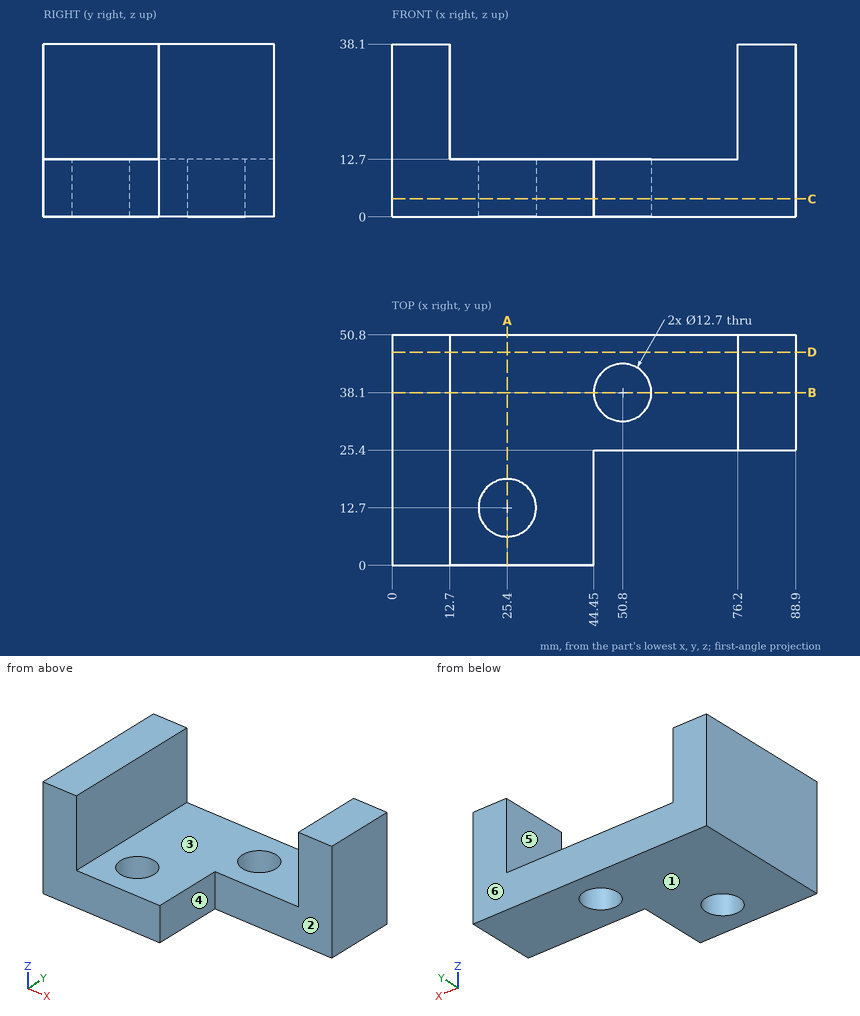
Job drawing, mm, ordinate dimensions from the low corner. One solid piece. A direction names the side the tool comes from. Coordinates: 2 decimals unless noted, no trailing zeros. Order: outer loops, then holes, each group sorted by start corner. A loop starts at its lowest first (then second) coordinate and runs counter-clockwise, first axis right, second up. Notation, with made-up numbers: (-11, 45) -> (32, 45) arc R11 cw to (32, 60) -> close; hole circle Ø8 at (30, -28.5). An arc over 180 degrees is marked (long way). Answer in a Markdown table with one row per item. Add a question column.
Q1. Band-saw the part on B-B, the plane y = 38.1. List the corners of the cut face in (x, z), then the cut area to 3 significant figures.
Q2. Band-saw the part on D-D, the plane y = 47. List the corners of the cut face in (x, z).
Q3. Wall check: line 1 along X through (y, z) = (34.5, 29.5); line 2 along Y through (x, z) = (50.8, 3.75); line 3 along Y through (x, z) = (25, 9). Give the ranges that are in metal, low to high. Write a range as [from, to].
Q4. Band-saw the part on C-C, the plane z = 4. List the corners of the cut face in (x, y).
Q5. Drop flat-ended pins along their axis: pin 1 (10 mm diameter, centred on x = 70.5, z = 33.5, fed in from +Y); pin 2 (1.5 mm diameter, centred on y = 12.5, z = 19.5, fed in from +X); pin 3 (19 mm diameter, centred on x = 76.5, z = 26.5, fed in from -Y); pin 4 (14 mm diameter, centred on y = 15.5, z = 6.5, fed in from +X). Give the stop position or say it passes through.
Q6. Mould opens along X. For the marked faces 4, 5 and 6 say: +X half, -X half, draft (parallel to the pull), parting line (faces both ways), or undercut.
Q7. Which spindle directions (+Z, -Z, +X, -X, +Y, -Y) get a long thin tool onto all of the face, cutting with end or side? Do the marked faces 1, 2 and 3. Say none if no direction does.
Q8. Band-saw the part on A-A, the plane x = 25.4. List the corners of the cut face in (y, z), then the cut area to 3 significant figures.
Answers follow:
| question | item | result |
|---|---|---|
| 1 | outline | (0, 0) -> (44.45, 0) -> (44.45, 12.7) -> (12.7, 12.7) -> (12.7, 38.1) -> (0, 38.1) -> close; (57.15, 0) -> (88.9, 0) -> (88.9, 38.1) -> (76.2, 38.1) -> (76.2, 12.7) -> (57.15, 12.7) -> close |
| 1 | area | 1,610 mm^2 |
| 2 | outline | (0, 0) -> (88.9, 0) -> (88.9, 38.1) -> (76.2, 38.1) -> (76.2, 12.7) -> (12.7, 12.7) -> (12.7, 38.1) -> (0, 38.1) -> close |
| 3 | line 1 | [0, 12.7], [76.2, 88.9] |
| 3 | line 2 | [25.4, 31.75], [44.45, 50.8] |
| 3 | line 3 | [0, 6.36], [19.04, 50.8] |
| 4 | outline | (0, 0) -> (44.45, 0) -> (44.45, 25.4) -> (88.9, 25.4) -> (88.9, 50.8) -> (0, 50.8) -> close; hole circle Ø12.7 at (25.4, 12.7); hole circle Ø12.7 at (50.8, 38.1) |
| 5 | pin 1 | through |
| 5 | pin 2 | x = 12.7 |
| 5 | pin 3 | y = 25.4 |
| 5 | pin 4 | x = 44.45 |
| 6 | face 4 | +X half |
| 6 | face 5 | undercut |
| 6 | face 6 | draft |
| 7 | face 1 | -Z, +X, -X, +Y, -Y |
| 7 | face 2 | +Z, -Z, +X, -Y |
| 7 | face 3 | +Z, +Y, -Y |
| 8 | outline | (0, 0) -> (6.35, 0) -> (6.35, 12.7) -> (0, 12.7) -> close; (19.05, 0) -> (50.8, 0) -> (50.8, 12.7) -> (19.05, 12.7) -> close |
| 8 | area | 484 mm^2 |
